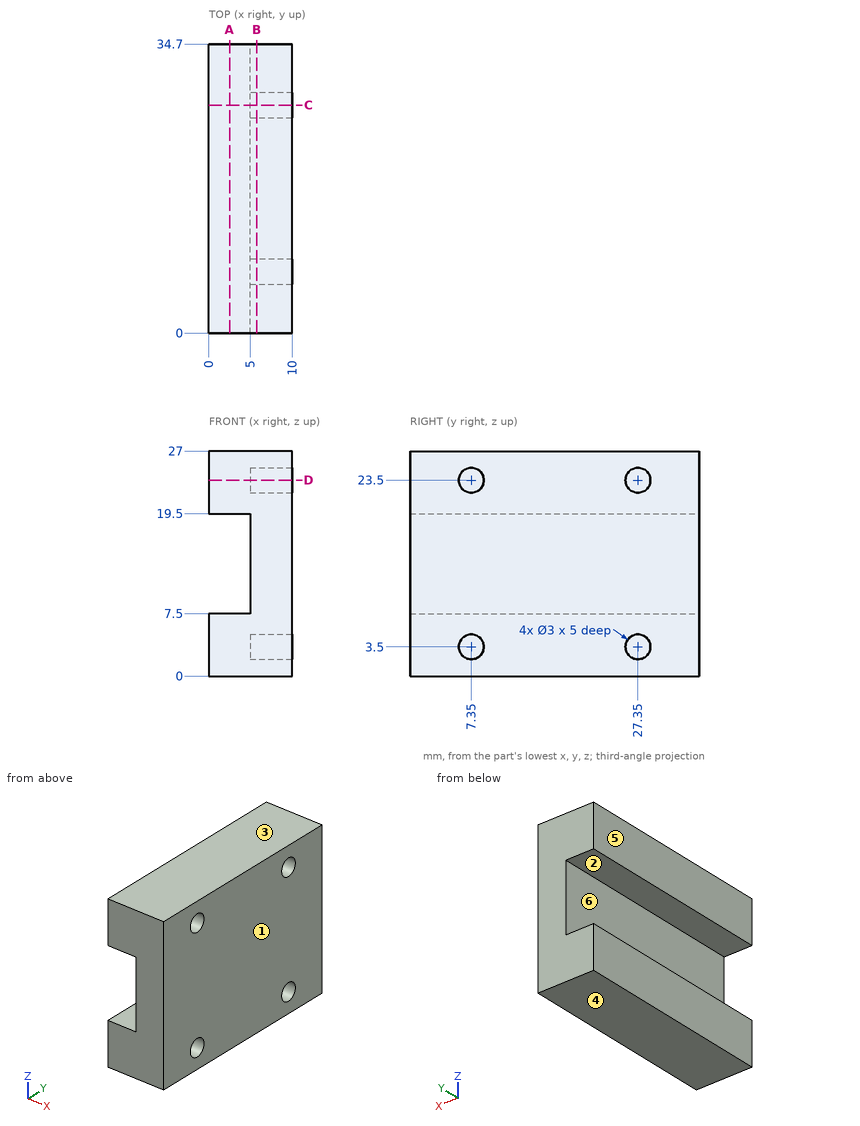
Design review of the part shown in the three views and the two pictorial views. Dimensions are in mm from the part's minimum x, y and z. A direction names the side the tool comes from. Round coordinates to 2 decimals unless told otherwise and drop trailing zeros. Loops run counter-clockwise (first coordinate to the right, second up) from the corner with the lowest first, then second, coordinate; pieces in that order, holes last. Notation, with made-up numbers: M 4,54.5 L 9,54.5 A20 cw 9,74.5 Z; hole C -15.75,47 d7. An arc over 180 degrees is marked long. Answer as a JSON object with one key per item and string values.
Item 1: We need section A-A, the plane x = 2.5. State the section outline as (y, z) points, and give its area (4 significant figures).
Check sheet entries:
{"outline": "M 0,0 L 34.7,0 L 34.7,7.5 L 0,7.5 Z; M 0,19.5 L 34.7,19.5 L 34.7,27 L 0,27 Z", "area": "520.5 mm2"}
Item 2: The part is to be moulded in two halves that separate along Z. For the marked faces 3, 4, 5 and 6, say which applies: +Z half, -Z half, draft (parallel to the pull), parting line (faces both ways), or undercut.
Check sheet entries:
{"face 3": "+Z half", "face 4": "-Z half", "face 5": "draft", "face 6": "undercut"}
Item 3: For line 1 along Z through (x, y) = (6.25, 27.35); line 2 along Y through (x, z) = (6.5, 23.5); line 3 along Z through (x, y) = (1.5, 14), list the stretches that pass through material, from the lowest coordinate up.
Check sheet entries:
{"line 1": "0 to 2, 5 to 22, 25 to 27", "line 2": "0 to 5.85, 8.85 to 25.85, 28.85 to 34.7", "line 3": "0 to 7.5, 19.5 to 27"}
Item 4: Clearance check with flat-ended pins moving along their axes: P1, Ø3.5, axis at y = 9.5, z = 13.5, coming from the -X side; P2, Ø2.5, axis at y = 7.35, z = 3.5, coming from the +X side; P3, Ø2, axis at x = 3.5, z = 14.5, coming from the -Y side. State where each tip first meets the part, or that it passes through.
Check sheet entries:
{"P1": "x = 5", "P2": "x = 5", "P3": "through"}
Item 5: We need section B-B, the plane x = 5.75. State the section outline as (y, z) points, and give its area (3 significant figures).
Check sheet entries:
{"outline": "M 0,0 L 34.7,0 L 34.7,27 L 0,27 Z; hole C 7.35,3.5 d3; hole C 7.35,23.5 d3; hole C 27.35,3.5 d3; hole C 27.35,23.5 d3", "area": "909 mm2"}
Item 6: We need section D-D, the plane z = 23.5. State the section outline as (x, y) points.
Check sheet entries:
{"outline": "M 0,0 L 10,0 L 10,5.85 L 5,5.85 L 5,8.85 L 10,8.85 L 10,25.85 L 5,25.85 L 5,28.85 L 10,28.85 L 10,34.7 L 0,34.7 Z"}
Item 7: We need section C-C, the plane y = 27.35. State the section outline as (x, z) points.
Check sheet entries:
{"outline": "M 0,0 L 10,0 L 10,2 L 5,2 L 5,5 L 10,5 L 10,22 L 5,22 L 5,25 L 10,25 L 10,27 L 0,27 L 0,19.5 L 5,19.5 L 5,7.5 L 0,7.5 Z"}
Item 8: Tool access review of the marked faces 1 and 2: name each direction out of +Z, -Z, +X, -X, +Y, -Y from which nothing blocks a thin tool from reaching the whole face with its end or side.
Check sheet entries:
{"face 1": "+Z, -Z, +X, +Y, -Y", "face 2": "-X, +Y, -Y"}
